CAD build for the part. Positions are in the model's coordinates, mm. Coordinates: 2 decimals unless noted, no trailing zeros. Loops run counter-clockwise (first coordinate to the right, second up) from the corner with the lowest first, then second, coordinate; pieces in that order, holes last. Notation, with made-up numbers: (-9, -25.75) -> (33, -25.75) arc R20 cw to (33, 12.25) -> close; hole circle Ø1 at (-27.75, 4). An arc over 180 degrees is marked (long way). Write item = value, one per line. Start each with the question number.
(1) Band-saw the part on A-A (x = -2.5). Write the cut outline in (y, z).
(2) Band-saw the part on B-B (z = 2.85). Count the separate pieces of the cut face and the enclosed holes in it, and give its area (3 significant figures).
(3) Flat gauge pins, fed straight in: P1, Ø3, axis at x = -51.5, z = 4.5, coming from the +Y side; P2, Ø1, axis at x = 74, z = 3.5, coming from the -Y side; P3, Ø1.8, axis at x = 38, z = 3.5, coming from the -Y side. Where does each tip first touch, or does it go through?
(4) Drill centre lines: line 1 (Y direction, x = 8, z = 4.5) (3 decimals); line 2 (X direction, y = -99, z = 5.6); line 3 (X direction, y = 96, z = 1.5). Where is each one in solid material? Low to high. Write a range as from..to.
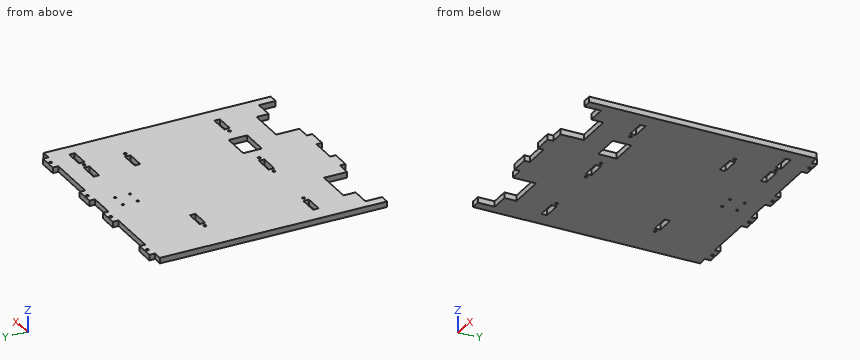
```python
from build123d import *

# Parameters (mm, degrees)
ESQUISSE1_W             = 218
ESQUISSE1_H             = 238
ESQUISSE1_W_2           = 20
ESQUISSE1_H_2           = 6
ESQUISSE1_W_3           = 30
ESQUISSE1_H_3           = 20
BOSS_EXTRU_1_DEPTH      = 6
ESQUISSE2_W             = 40
ESQUISSE2_H             = 25
ENL_V_MAT_EXTRU_1_DEPTH = 6
ESQUISSE3_W             = 20
ESQUISSE3_H             = 6
BOSS_EXTRU_3_DEPTH      = 6
ESQUISSE4_R             = 1.5
ENL_V_MAT_EXTRU_2_DEPTH = 6
ESQUISSE5_W             = 10
ESQUISSE5_H             = 244
BOSS_EXTRU_4_DEPTH      = 6
ESQUISSE6_W             = 20
ESQUISSE6_H             = 12
ENL_V_MAT_EXTRU_3_DEPTH = 6
ESQUISSE7_R             = 1.175
ENL_V_MAT_EXTRU_4_DEPTH = 7


with BuildPart() as part:
    # Esquisse1 → Boss.-Extru.1 (new body)
    with BuildSketch(Plane.XY):
        Rectangle(ESQUISSE1_W, ESQUISSE1_H)
        with Locations((-91, -58)):
            Rectangle(ESQUISSE1_W_2, ESQUISSE1_H_2, mode=Mode.SUBTRACT)
        with Locations((0, -58)):
            Rectangle(ESQUISSE1_W_2, ESQUISSE1_H_2, mode=Mode.SUBTRACT)
        with Locations((91, -58)):
            Rectangle(ESQUISSE1_W_2, ESQUISSE1_H_2, mode=Mode.SUBTRACT)
        with Locations((-66.5, 51)):
            Rectangle(ESQUISSE1_W_2, ESQUISSE1_H_2, mode=Mode.SUBTRACT)
        with Locations((66.5, 51)):
            Rectangle(ESQUISSE1_W_2, ESQUISSE1_H_2, mode=Mode.SUBTRACT)
        with Locations((45.5, -59)):
            Rectangle(ESQUISSE1_W_3, ESQUISSE1_H_3, mode=Mode.SUBTRACT)
        with Locations((65, 96)):
            Rectangle(ESQUISSE1_W_2, ESQUISSE1_H_2, mode=Mode.SUBTRACT)
        with Locations((95, 96)):
            Rectangle(ESQUISSE1_W_2, ESQUISSE1_H_2, mode=Mode.SUBTRACT)
    extrude(amount=BOSS_EXTRU_1_DEPTH)

    # Esquisse2 → Enlèv. mat.-Extru.1 (cut)
    with BuildSketch(Plane.XY.offset(6)):
        with Locations((-69, -106.5)):
            Rectangle(ESQUISSE2_W, ESQUISSE2_H)
        with Locations((69, -106.5)):
            Rectangle(ESQUISSE2_W, ESQUISSE2_H)
    extrude(amount=-ENL_V_MAT_EXTRU_1_DEPTH, mode=Mode.SUBTRACT)

    # Esquisse3 → Boss.-Extru.3 (add)
    with BuildSketch(Plane.XY.offset(6)):
        with Locations((-24, -122)):
            Rectangle(ESQUISSE3_W, ESQUISSE3_H)
        with Locations((24, -122)):
            Rectangle(ESQUISSE3_W, ESQUISSE3_H)
        with Locations((24, 122)):
            Rectangle(ESQUISSE3_W, ESQUISSE3_H)
        with Locations((99, 122)):
            Rectangle(ESQUISSE3_W, ESQUISSE3_H)
        with Locations((-24, 122)):
            Rectangle(ESQUISSE3_W, ESQUISSE3_H)
        with Locations((-99, 122)):
            Rectangle(ESQUISSE3_W, ESQUISSE3_H)
    extrude(amount=-BOSS_EXTRU_3_DEPTH)

    # Esquisse4 → Enlèv. mat.-Extru.2 (cut)
    with BuildSketch(Plane.XY.offset(6)):
        with Locations((-15, -58)):
            Circle(ESQUISSE4_R)
        with Locations((-76, -58)):
            Circle(ESQUISSE4_R)
        with Locations((80, 96)):
            Circle(ESQUISSE4_R)
        with Locations((81.5, 51)):
            Circle(ESQUISSE4_R)
        with Locations((76, -58)):
            Circle(ESQUISSE4_R)
        with Locations((15, -58)):
            Circle(ESQUISSE4_R)
        with Locations((-81.5, 51)):
            Circle(ESQUISSE4_R)
        with Locations((-99, 122)):
            Circle(ESQUISSE4_R)
        with Locations((-24, 122)):
            Circle(ESQUISSE4_R)
        with Locations((24, 122)):
            Circle(ESQUISSE4_R)
        with Locations((99, 122)):
            Circle(ESQUISSE4_R)
    extrude(amount=-ENL_V_MAT_EXTRU_2_DEPTH, mode=Mode.SUBTRACT)

    # Esquisse5 → Boss.-Extru.4 (add)
    with BuildSketch(Plane.XY.offset(6)):
        with Locations((-114, -3)):
            Rectangle(ESQUISSE5_W, ESQUISSE5_H)
        with Locations((114, -3)):
            Rectangle(ESQUISSE5_W, ESQUISSE5_H)
    extrude(amount=-BOSS_EXTRU_4_DEPTH)

    # Esquisse6 → Enlèv. mat.-Extru.3 (cut)
    with BuildSketch(Plane.XY.offset(6)):
        with Locations((99, -113)):
            Rectangle(ESQUISSE6_W, ESQUISSE6_H)
        with Locations((-99, -113)):
            Rectangle(ESQUISSE6_W, ESQUISSE6_H)
    extrude(amount=-ENL_V_MAT_EXTRU_3_DEPTH, mode=Mode.SUBTRACT)

    # Esquisse7 → Enlèv. mat.-Extru.4 (cut, through all)
    with BuildSketch(Plane.XY.offset(6)):
        with Locations((-8, 100.5)):
            Circle(ESQUISSE7_R)
        with Locations((8, 100.5)):
            Circle(ESQUISSE7_R)
        with Locations((-8, 84.5)):
            Circle(ESQUISSE7_R)
        with Locations((8, 84.5)):
            Circle(ESQUISSE7_R)
    extrude(amount=-ENL_V_MAT_EXTRU_4_DEPTH, mode=Mode.SUBTRACT)


solid = part.part
```
Findings below:
q1.outline = (-119, 0) -> (-61, 0) -> (-61, 6) -> (-119, 6) -> close; (-55, 0) -> (119, 0) -> (119, 6) -> (-55, 6) -> close
q2.separate_pieces = 1
q2.enclosed_holes = 23
q2.area = 53,500 mm²
q3.P1 = 119
q3.P2 = -94
q3.P3 = -119
q4.line_1 = -119..-61, -55..83.325, 85.675..99.325, 101.675..119
q4.line_2 = -119..-89, -49..49, 89..119
q4.line_3 = -119..55, 75..78.5, 81.5..85, 105..119
